Verification items for the finished model (mm, model axes). A direction names the side the tool comes from. Coordinates: 2 decimals unless noted, no trailing zeros. Order: outer loops, then holes, each group sorted by start corner. A loop starts at its lowest first (then second) coordinate and runs counter-clockwise, first axis right, second up. Notation, with made-up numbers: M -38.5,38.25 L 5.5,38.25 A20 cw 5.5,62.25 Z; hole C -31,67.5 d11. An arc over 180 degrees is marked long. Write item = value, one per line.
Autodesk Inventor part; units mm, degrees
ref_plane "Work Plane1" through (50.7701, 0, 0) normal (0, 0, -1) x (1, 0, 0)
ref_plane "YZ Plane" through (0, 0, 0) normal (1, 0, 0) x (0, 1, 0)
ref_plane "XZ Plane" through (0, 0, 0) normal (0, 1, 0) x (-1, 0, 0)
sketch "Sketch1" plane through (0, 0, 0) normal (0, 0, 1) x (1, 0, 0)
  line L0 (0, 0) -> (11.938, 0)
  line L1 (0, 0) -> (0, 8.001)
  line L2 (11.938, 7.493) -> (11.938, 0)
  line L3 (0, 8.001) -> (7.1937, 18.6779)
  line L4 (11.938, 7.493) -> (13.1445, 7.493)
  arc A0 (13.1445, 7.493) -> (7.1937, 18.6779) centre (13.1445, 14.6685) ccw
  line L5 (11.938, 7.493) -> (0, 8.001)
  line L6 (11.938, 7.493) -> (0, 7.493)
  dimension "d0" = 14.986
  dimension "d1" = 13.1445
  dimension "d2" = 14.6685
  dimension "d3" = 7.1755
  dimension "d4" = 11.938
  dimension "d5" = 16.002
revolve "Body" add sketch "Sketch1" angle 360 about axis through (0, 0, 0) along (1, 0, 0) contours L1 L6 L2 L0 | L1 L5 L6
extrude "Wing1" add sketch "Sketch1" along normal mid plane 5.08 contours L1 L5 L6 | L5 L3 A0 L4
fillet "Fillet1" [suppressed]
mirror "Wing2" about plane through (0, 0, 0) normal (0, 1, 0) of "Wing1"
sketch "Sketch2" plane through (0, 0, 0) normal (1, 0, 0) x (0, 1, 0)
  line L0 (0, -14) -> (0, 14)
  line L1 (-14, 0) -> (14, 0)
  point P0 (0, 0)
hole "Thread" at (0, 0, 0) direction (1, 0, 0) diameter 7.7978 end through all
chamfer "Chamfer1" distance 0.8593 angle 30 1 edges at (0, 0, -3.8989) measured on face at (0, 6.3482, -0.1567)
ref_plane "Work Plane1" through (50.7701, 0, 0) normal (0, 0, -1) x (1, 0, 0)
equation "\"d0\" = KOD2"
equation "\"d1\" = KOH1 - RR"
equation "\"d2\" = 0.5 * E0 - RR"
equation "\"d3\" = RR"
equation "\"d4\" = KOH"
equation "\"d5\" = KOD"
equation "\"d6\" = SW"
equation "\"d8\" = 0.333333 * SW"
equation "\"d9\" = -0.5 * GD1 + 0.5 * NND"
equation "\"d109\" = -0.5 * GD1 + 0.5 * NND"
equation "\"NND\" = 9.525"
equation "\"KOH\" = 11.938"
equation "\"KOH1\" = 20.32"
equation "\"SW\" = 5.08"
equation "\"KOD\" = 16.002"
equation "\"KOD2\" = 14.986"
equation "\"RR\" = 7.1755"
equation "\"E0\" = 43.688"
equation "\"THREADDIA\" = 9.525"
equation "\"TOA\" = 30deg"
equation "\"RR2\" = 2.8702"
equation "\"SW1\" = SW"
properties part number "ANSI B18.17 - 3/8 - 16" material "Steel, Mild"
Item 1: Sectioned sample at A-A, the plane y = 0. Enter the section's corners in (x, z).
Report:
outline = M 0,-8 L 11.94,-7.49 L 11.94,-3.9 L 0.5,-3.9 L 0,-4.76 Z; M 0,4.76 L 0.5,3.9 L 11.94,3.9 L 11.94,7.49 L 0,8 Z
Item 2: Sectioned sample at B-B, the plane x = 16. Enter the section's corners in (y, z).
Report:
outline = M -21.25,-2.54 L -8.09,-2.54 L -8.09,2.54 L -21.25,2.54 Z; M 8.09,-2.54 L 21.25,-2.54 L 21.25,2.54 L 8.09,2.54 Z
Item 3: Release check for a two-part mould opening along Y. For faces 4 (the cylindrical face through (19.574, -17.855, -0.036)), 5 (the flat face through (12, 13, -2.54)), 6 (the flat face through (3.546, 13.265, -0.036)) record: pulls with the +Y half, pulls with the -Y half, needs draft (parallel to the pull), parting line crosses it, or undercut.
Report:
face_4 = undercut
face_5 = needs draft
face_6 = pulls with the +Y half
Item 4: Sectioned sample at C-C, the plane x = 9.25. Enter the section's corners in (y, z).
Report:
outline = M -20.7,-2.54 L -7.49,-2.54 L -7.49,-1.31 A7.61 ccw 7.49,-1.31 L 7.49,-2.54 L 20.7,-2.54 L 20.7,2.54 L 7.49,2.54 L 7.49,1.31 A7.61 ccw -7.49,1.31 L -7.49,2.54 L -20.7,2.54 Z; hole C 0,0 d7.8
Item 5: Gauge pin test, flat ends, axial feed: pin 1 (7 mm diameter, centred on x = 11.5, y = 14.5, fed in from +Z); pin 2 (4 mm diameter, centred on x = 5, z = -1, fed in from -Y); pin 3 (10 mm diameter, centred on x = 6, y = -3, fed in from +Z). Record the tip position at first contact, or that the pin passes through.
Report:
pin_1 = 2.54
pin_2 = -18.39
pin_3 = 7.92
Item 6: Sectioned sample at D-D, the plane y = -9.5. Enter the section's corners in (x, z).
Report:
outline = M 1.01,-2.54 L 18.12,-2.54 L 18.12,2.54 L 1.01,2.54 Z
Item 7: Scan lines: L1, parallel to Z at x = 9, y = -12; L2, parallel to Y at x = 4.5, z = 0; L3, parallel to X at y = -6, z = -0.25. Record each from-to range of solid material in increasing order. Write a range as from..to.
Report:
L1 = -2.54..2.54
L2 = -14.68..-3.9, 3.9..14.68
L3 = 0..11.94
Item 8: Tool access check on faces 1 (the flat face through (11.938, 3, -3)), 2 (the flat face through (13, -15, 2.54)), 3 (the cylindrical face through (6.297, 2.372, -3.094)). Record the directions out of +Z, -Z, +X, -X, +Y, -Y that give a thin tool (end or side, any length) a straight path to the whole face; none if there is none.
Report:
face_1 = +Z, -Z, +X
face_2 = +Z, +X, -X, -Y
face_3 = +X, -X
